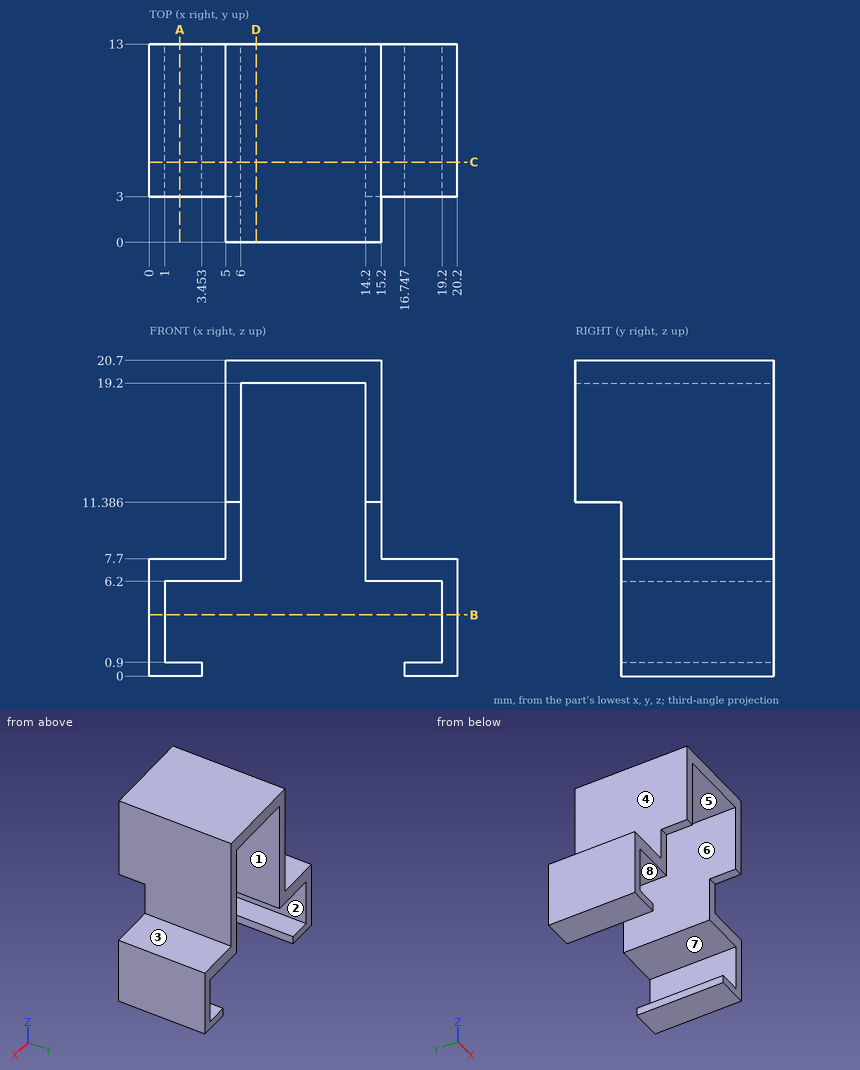
Geometry check sheet. Reference: drawing and pictorial views, mm from the part's lowest x, y, z. A direction names the side the tool comes from. Coordinates: 2 decimals unless noted, no trailing zeros. Order: outer loops, then holes, each group sorted by start corner. A loop starts at its lowest first (then second) coordinate and runs counter-clockwise, first axis right, second up. Notation, with made-up numbers: (46.5, 38.25) -> (53.5, 38.25) arc R5 ccw to (53.5, 47.25) -> close; hole circle Ø1 at (39.5, 84.5). An arc over 180 degrees is marked (long way). Use CSV: the item, a comma, the result in double quotes. Start each with the question number.
Q1. Section check B-B, the plane z = 4. Record the cut outline in (x, y).
Q2. Depth check by flat-ended pin: P1, Ø1.5, axis at y = 7.5, z = 5, coming from the -X side; P2, Ø5, axis at x = 10, z = 16.5, coming from the -Y side; P3, Ø5, axis at y = 5.5, z = 14, coming from the -X side; P4, Ø0.7, axis at x = 18, y = 9.5, coming from the +Z side. Enter the tip coordinate at first touch or a pass-through.
Q3. Section check D-D, the plane x = 7. Record the cut outline in (y, z), and give its area (3 significant figures).
Q4. Draft check along Z on the marked faces 5, 6, 7 and 8. Enter one of: +Z half, -Z half, draft (parallel to the pull), parting line (faces both ways), or undercut.
Q5. Section check A-A, the plane x = 2. Record the cut outline in (y, z), and give its area (3 significant figures).
Q6. Tool access check on the marked faces 1, 2, 3 and 4. Record the directions out of +Z, -Z, +X, -X, +Y, -Y that give a thin tool (end or side, any length) a straight path to the whole face; none if there is none.
Q7. Thickness scan on line 1 along X through (y, z) = (12.25, 14.5); line 2 along X through (y, z) = (6, 2); line 3 along Z through (x, y) = (19, 12). Record the ranges inside material, lowest first.
Q8. Section check C-C, the plane y = 5.25. Record the cut outline in (x, z).
Returned:
1,outline,"(0, 3) -> (1, 3) -> (1, 13) -> (0, 13) -> close; (19.2, 3) -> (20.2, 3) -> (20.2, 13) -> (19.2, 13) -> close"
2,P1,"stops at x = 0"
2,P2,"passes through"
2,P3,"stops at x = 5"
2,P4,"stops at z = 7.7"
3,outline,"(0, 19.2) -> (13, 19.2) -> (13, 20.7) -> (0, 20.7) -> close"
3,area,"19.5 mm^2"
4,face 5,"-Z half"
4,face 6,"draft"
4,face 7,"undercut"
4,face 8,"undercut"
5,outline,"(3, 0) -> (13, 0) -> (13, 0.9) -> (3, 0.9) -> close; (3, 6.2) -> (13, 6.2) -> (13, 7.7) -> (3, 7.7) -> close"
5,area,"24.0 mm^2"
6,face 1,"-Z, +Y, -Y"
6,face 2,"+Y, -Y"
6,face 3,"+Z, +X, +Y, -Y"
6,face 4,"+Z, -X, +Y, -Y"
7,line 1,"x = 5 to 6, 14.2 to 15.2"
7,line 2,"x = 0 to 1, 19.2 to 20.2"
7,line 3,"z = 0 to 0.9, 6.2 to 7.7"
8,outline,"(0, 0) -> (3.45, 0) -> (3.45, 0.9) -> (1, 0.9) -> (1, 6.2) -> (6, 6.2) -> (6, 19.2) -> (14.2, 19.2) -> (14.2, 6.2) -> (19.2, 6.2) -> (19.2, 0.9) -> (16.75, 0.9) -> (16.75, 0) -> (20.2, 0) -> (20.2, 7.7) -> (15.2, 7.7) -> (15.2, 20.7) -> (5, 20.7) -> (5, 7.7) -> (0, 7.7) -> close"
